Autodesk Inventor part; units mm, degrees
ref_plane "YZ Plane" through (0, 0, 0) normal (1, 0, 0) x (0, 1, 0)
ref_plane "XZ Plane" through (0, 0, 0) normal (0, 1, 0) x (-1, 0, 0)
ref_plane "XY Plane" through (0, 0, 0) normal (0, 0, 1) x (1, 0, 0)
sketch "Sketch1" plane through (0, 0, 0) normal (0, 0, 1) x (1, 0, 0)
  line L0 (-12.5, -15) -> (12.5, -15)
  line L1 (12.5, -15) -> (12.5, 15)
  line L2 (12.5, 15) -> (-12.5, 15)
  line L3 (-12.5, 15) -> (-12.5, -15)
  line L4 (-12.5, -15) -> (12.5, 15) construction
  line L5 (12.5, -15) -> (-12.5, 15) construction
  point P0 (0, 0)
  dimension "d0" = 30
  dimension "d1" = 25
extrude "Extrusion1" add sketch "Sketch1" along normal mid plane 5
sketch "Sketch2" plane through (0, 0, 2.5) normal (0, 0, 1) x (1, 0, 0)
  line L0 (-12.5, 15) -> (-12.5, -15)
  line L1 (12.5, 15) -> (-12.5, 15)
  point P0 (0, 0)
  point P1 (2.5, 7.5)
  point P2 (2.5, -7.5)
  dimension "d4" = 15
  dimension "d5" = 7.5
  dimension "d6" = 15
hole "Hole1" at (2.5, 7.5, 2.5) at (2.5, -7.5, 2.5) direction (0, 0, -1) diameter 7 depth 14.2 tip angle 118
properties part number "HCMUTE-CDT23-DE_CHEM_LOADCELL" material "PMMA Plastic"
The listing builds one solid part. Answer for the finished solid, in the listing's coordinates (mm). Coordinates: 2 decimals unless noted, no trailing zeros. Loops run counter-clockwise (first coordinate to the right, second up) from the corner with the lowest first, then second, coordinate; pieces in that order, holes last. Notation, with made-up numbers: (75, -33) -> (84, -33) arc R26 cw to (84, 3) -> close; hole circle Ø9 at (59, 76). An arc over 180 degrees is marked (long way). Return JSON: item names as keys, results as strings. Group by question number.
(1) Given pin 1 Ø5.5 at (x, y) = (2.5, 7.5) entering from +Z, flat-ended and moving along its own axis, determine where the tip first touches the part or whether it passes through.
(2) A cutting plane is placed at B-B on x = 2.5. Write down the section's boundary in (y, z), and give its area (3 significant figures).
(3) Find the intervals of material crossed by probe 1 along Y at (x, z) = (2.5, -0.9); probe 2 along X at (y, z) = (-7.5, -0.3); probe 3 along Y at (x, z) = (-0.25, 0.7), in increasing order. Write a range as from..to.
(4) A cutting plane is placed at C-C on z = -0.8. Write down the section's boundary in (x, y).
(5) A cutting plane is placed at A-A on y = -7.5. Write down the section's boundary in (x, z).
(6) A cutting plane is placed at D-D on y = 9.25. Write down the section's boundary in (x, z).
The answers:
{
 "1": {"pin 1": "passes through"},
 "2": {"outline": "(-15, -2.5) -> (-11, -2.5) -> (-11, 2.5) -> (-15, 2.5) -> close; (-4, -2.5) -> (4, -2.5) -> (4, 2.5) -> (-4, 2.5) -> close; (11, -2.5) -> (15, -2.5) -> (15, 2.5) -> (11, 2.5) -> close", "area": "80.0 mm^2"},
 "3": {"probe 1": "y = -15..-11, -4..4, 11..15", "probe 2": "x = -12.5..-1, 6..12.5", "probe 3": "y = -15..-9.67, -5.33..5.33, 9.67..15"},
 "4": {"outline": "(-12.5, -15) -> (12.5, -15) -> (12.5, 15) -> (-12.5, 15) -> close; hole circle Ø7 at (2.5, -7.5); hole circle Ø7 at (2.5, 7.5)"},
 "5": {"outline": "(-12.5, -2.5) -> (-1, -2.5) -> (-1, 2.5) -> (-12.5, 2.5) -> close; (6, -2.5) -> (12.5, -2.5) -> (12.5, 2.5) -> (6, 2.5) -> close"},
 "6": {"outline": "(-12.5, -2.5) -> (-0.53, -2.5) -> (-0.53, 2.5) -> (-12.5, 2.5) -> close; (5.53, -2.5) -> (12.5, -2.5) -> (12.5, 2.5) -> (5.53, 2.5) -> close"}
}
